```python
from build123d import *

# Parameters (mm, degrees)
BOSS_EXTRUDE1_DEPTH  = 50
M6_CLEARANCE_HOLE1_D = 6.4


with BuildPart() as part:
    # Sketch1 → Boss-Extrude1 (new body)
    with BuildSketch(Plane.XY):
        Polygon((0, 0), (0, 4.5), (5.5, 4.5), (5.5, 19), (28.5, 19), (28.5, 4.5), (34, 4.5), (34, 0), (23.25, 0), (23.25, 3.75), (10.75, 3.75), (10.75, 0), align=None)
    extrude(amount=BOSS_EXTRUDE1_DEPTH)

    # M6 Clearance Hole1 (through all)
    with Locations(Plane(origin=(17, 19, 15), x_dir=(0, 0, 1), z_dir=(0, 1, 0))):
        with Locations((0, 0), (20, 0)):
            Hole(M6_CLEARANCE_HOLE1_D / 2)


solid = part.part
```
CAD build for the part. Positions are in the model's coordinates, mm. A direction names the side the tool comes from. Coordinates: 2 decimals unless noted, no trailing zeros. Order: outer loops, then holes, each group sorted by start corner. A loop starts at its lowest first (then second) coordinate and runs counter-clockwise, first axis right, second up.
(1) Saw through at B-B, the plane x = 17. Write the cut outline in (y, z).
Solution:
outline: (3.75, 0) - (19, 0) - (19, 11.8) - (3.75, 11.8) - close; (3.75, 18.2) - (19, 18.2) - (19, 31.8) - (3.75, 31.8) - close; (3.75, 38.2) - (19, 38.2) - (19, 50) - (3.75, 50) - close
(2) Drill centre lines: L1, parallel to X at y = 13.25, z = 15; L2, parallel to X at y = 7.5, z = 20; L3, parallel to Y at x = 20, z = 2. Where is each one in solid material? Low to high.
Solution:
L1: x = 5.5 to 13.8, 20.2 to 28.5
L2: x = 5.5 to 28.5
L3: y = 3.75 to 19
(3) Mould opens along X. For faces 1 (the face through (17, 10, 50)), 2 (the face through (5.5, 12, 25)), 3 (the face through (13.876, 11.268, 15.694)) say: released by +X, released by -X, zero draft, split by the parting line, or undercut.
Solution:
face 1: zero draft
face 2: released by -X
face 3: undercut
(4) Saw through at A-A, the plane z = 35. Write the cut outline in (x, y), and give its area (3 significant figures).
Solution:
outline: (0, 0) - (10.75, 0) - (10.75, 3.75) - (13.8, 3.75) - (13.8, 19) - (5.5, 19) - (5.5, 4.5) - (0, 4.5) - close; (20.2, 3.75) - (23.25, 3.75) - (23.25, 0) - (34, 0) - (34, 4.5) - (28.5, 4.5) - (28.5, 19) - (20.2, 19) - close
area: 342 mm2
(5) Saw through at C-C, the plane z = 44.5. Write the cut outline in (x, y), and give its area (3 significant figures).
Solution:
outline: (0, 0) - (10.75, 0) - (10.75, 3.75) - (23.25, 3.75) - (23.25, 0) - (34, 0) - (34, 4.5) - (28.5, 4.5) - (28.5, 19) - (5.5, 19) - (5.5, 4.5) - (0, 4.5) - close
area: 440 mm2
(6) Saw through at D-D, the plane y = 15.75. Write the cut outline in (x, z).
Solution:
outline: (5.5, 0) - (28.5, 0) - (28.5, 50) - (5.5, 50) - close; hole circle Ø6.4 at (17, 15); hole circle Ø6.4 at (17, 35)
(7) Which spindle directions (+Z, -Z, +X, -X, +Y, -Y) get a long thin tool onto all of the face, cutting with end or side? Do faces 4 (the face through (10.75, 2, 25)), 5 (the face through (3, 4.5, 25)), 6 (the face through (31, 4.5, 25)). Say none if no direction does.
Solution:
face 4: +Z, -Z, -Y
face 5: +Z, -Z, -X, +Y
face 6: +Z, -Z, +X, +Y
(8) Pin check, flat tips, straight feed: pin 1 Ø8.5 at (x, z) = (17, 15) entering from +Y; pin 2 Ø10 at (x, z) = (17.5, 22) entering from -Y; pin 3 Ø5 at (y, z) = (10, 30) entering from +X; pin 4 Ø1.6 at (x, z) = (32, 18.5) entering from +Y. Stop position of each tip, or through.
Solution:
pin 1: stops at y = 19
pin 2: stops at y = 3.75
pin 3: stops at x = 28.5
pin 4: stops at y = 4.5
